Geometry: final body of the model. Coordinates: model frame, mm. A direction names the side the tool comes from. Round coordinates to 2 decimals unless told otherwise and drop trailing zeros. Loops run counter-clockwise (first coordinate to the right, second up) from the corner with the lowest first, then second, coordinate; pieces in that order, holes last. Notation, with made-up numbers: M 72.5,2.5 L 84.5,2.5 A21 cw 84.5,33.5 Z; hole C 3,-14.75 d11. An arc over 180 degrees is marked long. Answer as a JSON object with one key per item and string values.
Autodesk Inventor part; units mm, degrees
ref_plane "YZ Plane" through (0, 0, 0) normal (1, 0, 0) x (0, 1, 0)
ref_plane "XZ Plane" through (0, 0, 0) normal (0, 1, 0) x (-1, 0, 0)
ref_plane "XY Plane" through (0, 0, 0) normal (0, 0, 1) x (1, 0, 0)
sketch "Boceto1" plane through (0, 0, 0) normal (0, 1, 0) x (-1, 0, 0)
  line L0 (-6.5, -6.5) -> (6.5, -6.5)
  line L1 (6.5, -6.5) -> (6.5, 6.5)
  line L2 (6.5, 6.5) -> (-6.5, 6.5)
  line L3 (-6.5, 6.5) -> (-6.5, -6.5)
  line L4 (-6.5, -6.5) -> (6.5, 6.5) construction
  line L5 (6.5, -6.5) -> (-6.5, 6.5) construction
  point P0 (0, 0)
  dimension "d0" = 13
  dimension "d1" = 13
extrude "Extrusión1" add sketch "Boceto1" along normal blind 13
shell "Vaciado1" thickness 1.5 removed faces 2 at (6.5, 4.3333, 2.1667) at (-2.1667, 13, -2.1667)
chamfer "Chaflán1" distance 11.5 angle 45 2 edges at (6.5, 13, 5.75) (6.5, 13, -5.75)
sketch "Boceto2" plane through (0, 0, 0) normal (0, -1, 0) x (1, 0, 0)
  line L0 (-6.5, 6.5) -> (6.5, 6.5)
  line L1 (-6.5, -6.5) -> (-6.5, 6.5)
  point P0 (0, 0)
  point P1 (0, 0)
  dimension "d8" = 6.5
  dimension "d9" = 6.5
hole "Agujero1" at (0, 0, 0) direction (0, 1, 0) diameter 3 depth 3 tip angle 118
sketch "Boceto3" plane through (-6.5, 0, -6.5) normal (-1, 0, 0) x (0, 0, 1)
  line L0 (0, 0) -> (13, 0)
  line L1 (13, 0) -> (13, 13)
  point P0 (6.5, 0)
  point P1 (6.5, 6.5)
  dimension "d17" = 6.5
  dimension "d18" = 6.5
hole "Agujero2" at (-6.5, 6.5, 0) direction (1, 0, 0) diameter 3 depth 3 tip angle 118
properties part number "Escuadra"
1) Section query D-D (y = 9). Return the cut outline in (x, z), and give its area (3 significant figures).
Results:
{"outline": "M -6.5,-6.5 L -1,-6.5 L -1,-5 L -5,-5 L -5,5 L -1,5 L -1,6.5 L -6.5,6.5 Z", "area": "31.5 mm2"}
2) Section query A-A (x = 0). Return the cut outline in (y, z).
Results:
{"outline": "M 0,-6.5 L 8,-6.5 L 8,-5 L 1.5,-5 L 1.5,-1.5 L 0,-1.5 Z; M 0,1.5 L 1.5,1.5 L 1.5,5 L 8,5 L 8,6.5 L 0,6.5 Z"}
3) Section query B-B (z = -0.5). Return the cut outline in (x, y), and give its area (3 significant figures).
Results:
{"outline": "M -6.5,0 L -1.41,0 L -1.41,1.5 L -5,1.5 L -5,5.09 L -6.5,5.09 Z; M -6.5,7.91 L -5,7.91 L -5,13 L -6.5,13 Z; M 1.41,0 L 6.5,0 L 6.5,1.5 L 1.41,1.5 Z", "area": "28.3 mm2"}
4) Pin query (flat end, axial travel): P1, Ø4, axis at x = 2, z = 0.5, coming from the +Y side; P2, Ø1.5, axis at x = 0, y = 11, coming from the +Z side; P3, Ø3, axis at y = 6, z = 2, coming from the +X side; P4, Ø4, axis at x = 3.5, z = -3.5, coming from the +Y side. Return the tip coordinate at first contact, or that it passes through.
Results:
{"P1": "y = 1.5", "P2": "through", "P3": "x = -5", "P4": "y = 5.82"}
5) Section query C-C (y = 6.5). Return the cut outline in (x, z), and give its area (3 significant figures).
Results:
{"outline": "M -6.5,-6.5 L 1.5,-6.5 L 1.5,-5 L -5,-5 L -5,-1.5 L -6.5,-1.5 Z; M -6.5,1.5 L -5,1.5 L -5,5 L 1.5,5 L 1.5,6.5 L -6.5,6.5 Z", "area": "34.5 mm2"}
6) Reachability of faces 4 (the flat face through (-6, 13, 0)), 5 (the flat face through (2, 1.5, 0)) from +Z, -Z, +X, -X, +Y, -Y: full face, straight path, thin tool, end or side. Return the list, or none.
Results:
{"face 4": "+Z, -Z, +X, -X, +Y", "face 5": "+X, +Y"}
7) Ray query, line 1 (Z direction, x = 0, y = 1); line 2 (Z direction, x = -2.75, y = 10). Return the intervals inside material, ascending.
Results:
{"line 1": "-6.5 to -1.5, 1.5 to 6.5", "line 2": "-6.5 to -5, 5 to 6.5"}
8) Pull-direction query (Z, two-part tool) for faces 1 (the flat face through (-2, 5, -5)), 2 (the flat face through (6.5, 1, 0)), 3 (the flat face through (-2, 5, 6.5)); classes: +Z half, -Z half, draft (parallel to the pull), parting line (faces both ways), or undercut.
Results:
{"face 1": "undercut", "face 2": "draft", "face 3": "+Z half"}
